Part print with two shaded views. Sizes in mm from the minimum x, y, z corner. Coordinates: 2 decimals unless noted, no trailing zeros. Loops run counter-clockwise (first coordinate to the right, second up) from the corner with the lowest first, then second, coordinate; pieces in that order, holes last. Notation, with made-up numbers: (75.25, 8.25) -> (99.25, 8.25) arc R15 ccw to (99.25, 23.25) -> close; hole circle Ø4 at (4, -11). An arc over 180 degrees is marked (long way). One line per item, written item: value. Start each with the question number.
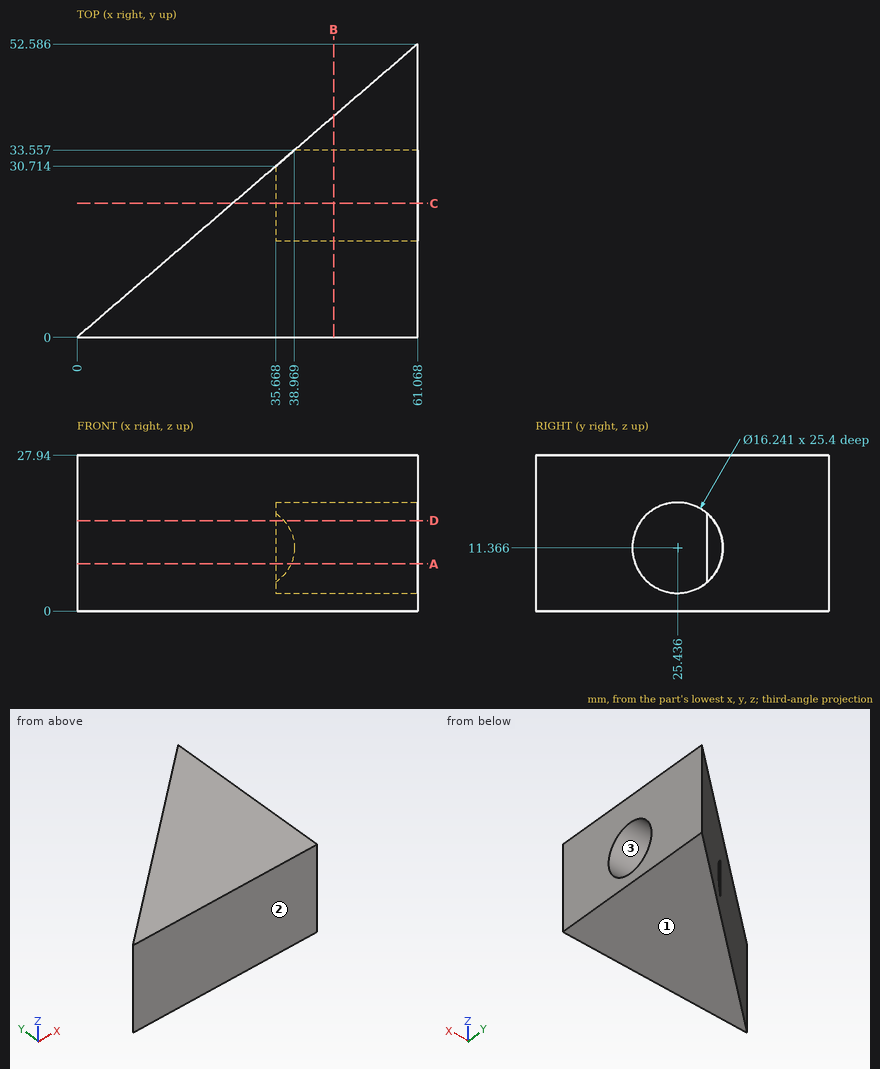
Item 1: Drop flat-ended pins along their axis: pin 1 Ø14.5 at (y, z) = (25.44, 11.37) entering from +X; pin 2 Ø5 at (x, z) = (51.5, 19) entering from +Y; pin 3 Ø4 at (y, z) = (22.5, 10.5) entering from -X (1 decimal). Give the stop position or say it passes through.
Item 2: Band-saw the part on B-B, the plane x = 46. List the corners of the cut face in (y, z).
Item 3: Two-plate mould, pull along Z, no slides. Class the marked faces 1, 2 and 3: +Z half, -Z half, draft (parallel to the pull), parting line (faces both ways), or undercut.
Item 4: Band-saw the part on C-C, the plane y = 24. List the corners of the cut face in (x, z).
Item 5: Probe probe 1 along Y at (x, z) = (49, 18) (1 decimal); probe 2 along Z at (x, y) = (53, 31); probe 3 along Y at (x, z) = (38.5, 7) (1 decimal). List the from-to ranges inside material, lowest first.
Item 6: Band-saw the part on A-A, the plane z = 8.5. List the corners of the cut face in (x, y) (1 decimal).
Item 7: Band-saw the part on D-D, the plane z = 16.25. List the corners of the cut face in (x, y), and give its area (3 significant figures).
Worked out:
1. pin 1: stops at x = 35.67
1. pin 2: stops at y = 46.5
1. pin 3: stops at x = 23.8
2. outline: (0, 0) -> (39.61, 0) -> (39.61, 27.94) -> (0, 27.94) -> close; hole circle Ø16.24 at (25.44, 11.37)
3. face 1: -Z half
3. face 2: draft
3. face 3: undercut
4. outline: (27.87, 0) -> (61.07, 0) -> (61.07, 3.37) -> (35.67, 3.37) -> (35.67, 19.36) -> (61.07, 19.36) -> (61.07, 27.94) -> (27.87, 27.94) -> close
5. probe 1: y = 0 to 20.8, 30.1 to 42.2
5. probe 2: z = 0 to 5.45, 17.28 to 27.94
5. probe 3: y = 0 to 18.6, 32.3 to 33.2
6. outline: (0, 0) -> (61.1, 0) -> (61.1, 17.8) -> (35.7, 17.8) -> (35.7, 30.7) -> close; (38.4, 33) -> (61.1, 33) -> (61.1, 52.6) -> close
7. outline: (0, 0) -> (61.07, 0) -> (61.07, 18.95) -> (35.67, 18.95) -> (35.67, 30.71) -> close; (37.07, 31.92) -> (61.07, 31.92) -> (61.07, 52.59) -> close
7. area: 1,280 mm²
